Geometry: final body of the model. Coordinates: model frame, mm. Face numbers are marked on the shaded views. Give positions to 0.01 mm unless a question says otherwise; leave off trailing zeros. Write each loop counter-clockwise with the first axis right and the second up, starting at its lowest first coordinate (ties: lowest second). Pieces come first, ordered by that corner, then holes. Notation, with made-up numbers: M 89.25,48 L 96.25,48 A14 ccw 96.25,62 Z; hole C -9.75,4 d4. An arc over 180 degrees is marked long. Use a Markdown table: item, result. Add a question column.
(1) Cut plane B-B (x = 15.24). Output: boundary loops of the cut face in (y, z).
(2) Material intervals for L1, parallel to X at y = 3.25, z = -27.81; L2, parallel to Z at x = -15.5, y = 4; L3, parallel to X at y = 3, z = 21.59, sorted ascending.
(3) Cut plane A-A (z = -12.31). Output: boundary loops of the cut face in (x, y), plus the area to 3 significant figures.
(4) Cut plane C-C (z = -27.81). Output: boundary loops of the cut face in (x, y), plus the area to 3 significant figures.
(5) Draft query along Z for the marked faces 1, 2 and 3. Return one class per face: released by +Z, released by -Z, zero draft, split by the parting line, or undercut.
(6) Pin query (flat end, axial travel): pin 1 Ø2.5 at (x, z) = (-15.5, -27.81) entering from +Y. Return the tip coordinate at first contact, or that it passes through.
(7) Cut plane D-D (y = 3.5). Output: boundary loops of the cut face in (x, z), plus the area to 3 significant figures.
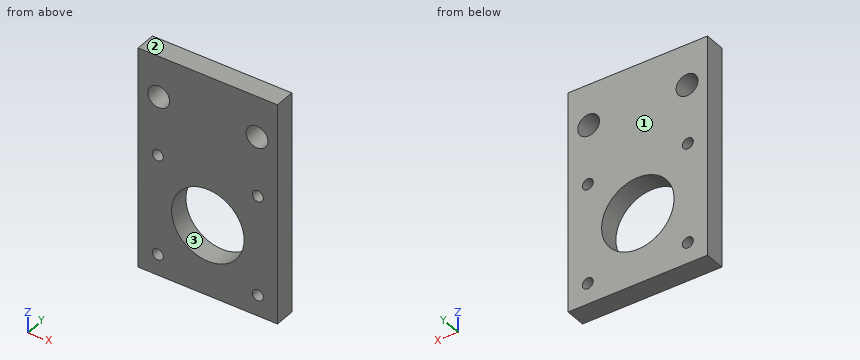
```python
from build123d import *

# Parameters (mm, degrees)
SKETCH1_W               = 43.18
SKETCH1_H               = 68.58
BOSS_EXTRUDE1_DEPTH     = 6.35
F_1_4_CLEARANCE_HOLE1_D = 6.7564
SKETCH7_R               = 11.239
CUT_EXTRUDE1_DEPTH      = 7.35
M3_CLEARANCE_HOLE1_D    = 3.4


with BuildPart() as part:
    # Sketch1 → Boss-Extrude1 (new body)
    with BuildSketch(Plane(origin=(0, 0, 0), x_dir=(1, 0, 0), z_dir=(0, 1, 0))):
        Rectangle(SKETCH1_W, SKETCH1_H)
    extrude(amount=BOSS_EXTRUDE1_DEPTH)

    # 1/4 Clearance Hole1 (through all)
    with Locations(Plane(origin=(0, 6.35, 0), x_dir=(1, 0, 0), z_dir=(0, 1, 0))):
        with Locations((15.24, -21.59), (-15.24, -21.59)):
            Hole(F_1_4_CLEARANCE_HOLE1_D / 2)

    # Sketch7 → Cut-Extrude1 (cut, through all)
    with BuildSketch(Plane.XZ):
        with Locations((0, -12.31)):
            Circle(SKETCH7_R)
    extrude(amount=-CUT_EXTRUDE1_DEPTH, mode=Mode.SUBTRACT)

    # M3 Clearance Hole1 (through all)
    with Locations(Plane(origin=(0, 0, 0), x_dir=(-1, 0, 0), z_dir=(0, -1, 0))):
        with Locations((-15.5, 27.81), (15.5, 27.81), (15.5, -3.19), (-15.5, -3.19)):
            Hole(M3_CLEARANCE_HOLE1_D / 2)


solid = part.part
```
Answer list:
| question | item | result |
|---|---|---|
| 1 | outline | M 0,-34.29 L 6.35,-34.29 L 6.35,-29.49 L 0,-29.49 Z; M 0,-26.13 L 6.35,-26.13 L 6.35,1.51 L 0,1.51 Z; M 0,4.87 L 6.35,4.87 L 6.35,18.21 L 0,18.21 Z; M 0,24.97 L 6.35,24.97 L 6.35,34.29 L 0,34.29 Z |
| 2 | L1 | -21.59 to -17.2, -13.8 to 13.8, 17.2 to 21.59 |
| 2 | L2 | -34.29 to -29.51, -26.11 to 1.49, 4.89 to 18.22, 24.96 to 34.29 |
| 2 | L3 | -21.59 to -18.62, -11.86 to 11.86, 18.62 to 21.59 |
| 3 | outline | M -21.59,0 L -11.24,0 L -11.24,6.35 L -21.59,6.35 Z; M 11.24,0 L 21.59,0 L 21.59,6.35 L 11.24,6.35 Z |
| 3 | area | 131 mm² |
| 4 | outline | M -21.59,0 L -17.2,0 L -17.2,6.35 L -21.59,6.35 Z; M -13.8,0 L 13.8,0 L 13.8,6.35 L -13.8,6.35 Z; M 17.2,0 L 21.59,0 L 21.59,6.35 L 17.2,6.35 Z |
| 4 | area | 231 mm² |
| 5 | face 1 | zero draft |
| 5 | face 2 | released by +Z |
| 5 | face 3 | undercut |
| 6 | pin 1 | through |
| 7 | outline | M -21.59,-34.29 L 21.59,-34.29 L 21.59,34.29 L -21.59,34.29 Z; hole C -15.24,21.59 d6.76; hole C -15.5,-27.81 d3.4; hole C -15.5,3.19 d3.4; hole C 0,-12.31 d22.48; hole C 15.24,21.59 d6.76; hole C 15.5,-27.81 d3.4; hole C 15.5,3.19 d3.4 |
| 7 | area | 2,460 mm² |
